CAD build for the part. Positions are in the model's coordinates, mm. Round coordinates to 2 decimals unless told otherwise and drop trailing zeros. Order: outer loops, then holes, each group sorted by start corner. A loop starts at its lowest first (then second) coordinate and runs counter-clockwise, first axis right, second up. Notation, with made-up numbers: (43, 42.25) - (52, 42.25) arc R24 ccw to (52, 64.25) - close; hole circle Ø10 at (31, -13.5). An arc over 180 degrees is marked (long way). Write item = value, one per line.
from build123d import *

# Parameters (mm, degrees)
SWEEP1_PROFILE_R    = 12.7
SKETCH2_R           = 25.4
BOSS_EXTRUDE1_DEPTH = 127
FILLET1_R           = 16.51


with BuildPart() as part:
    # Sweep1: sweep along a path in Sketch1
    with BuildLine(Plane.XY) as sweep1_path:
        Line((-127, 0), (-25.4, 0))
        ThreePointArc((-25.4, 0), (-7.439487758, 7.439487758), (0, 25.4))
        Line((0, 25.4), (0, 88.9))
    # Sweep1 profile (on start of the path) → Sweep1 (sweep)
    with BuildSketch(Plane.YZ.offset(-127)):
        Circle(SWEEP1_PROFILE_R)
    sweep(path=sweep1_path.line)

    # Sketch2 → Boss-Extrude1 (add)
    with BuildSketch(Plane(origin=(0, 88.9, 0), x_dir=(1, 0, 0), z_dir=(0, 1, 0))):
        with Locations(Location((0, 0, 0), (0, 0, 270))):
            Circle(SKETCH2_R)
    extrude(amount=BOSS_EXTRUDE1_DEPTH)

    # Fillet1
    # the kernel refuses this fillet: 16.51 mm, written as the material it takes off along each edge
    with BuildSketch(Plane(origin=(0, 88.9, 0), x_dir=(0, 0, 1), z_dir=(-1, 0, 0))) as fillet1_piece_1:
        with BuildLine():
            CenterArc((8.89, 16.064370514), FILLET1_R, 283.342363797, 76.657636203)
            Line((12.7, 0), (12.7762, -0.32128741))
            ThreePointArc((12.7762, -0.32128741), (19.05, -0.3302), (25.4, -0.3302))
            Line((25.4, -0.3302), (25.7302, 0))
            Line((25.7302, 0), (25.7302, 16.064370514))
            Line((25.7302, 16.064370514), (25.4, 16.064370514))
        make_face()
    revolve(axis=Axis((0, 88.9, 0), (0, 1, 0)), mode=Mode.SUBTRACT)


solid = part.part
(1) Probe line 1 along X through (y, z) = (140, -1); line 2 along Y through (x, z) = (-68.5, -1); line 3 along Y through (x, z) = (-69.5, 4). List the from-to ranges inside material, lowest first.
Solved:
line_1 = -25.38 to 25.38
line_2 = -12.66 to 12.66
line_3 = -12.05 to 12.05
(2) Drop flat-ended pins along their axis: pin 1 (5 mm diameter, centred on x = -63, z = 7, fed in from +Y); pin 2 (1.5 mm diameter, centred on x = -7.5, y = 160.5, fed in from +Z); pin 3 (2 mm diameter, centred on x = -45.5, z = 4, fed in from -Y). Give the stop position or say it passes through.
Solved:
pin_1 = 11.88
pin_2 = 24.49
pin_3 = -12.34
(3) Band-saw the part on B-B on x = -113. List the corners of the cut face in (y, z), plus the area to 3 significant figures.
Solved:
outline = circle Ø25.4 at (0, 0)
area = 507 mm²
(4) Band-saw the part on A-A on y = 112. List the corners of the cut face in (x, z).
Solved:
outline = circle Ø50.8 at (0, 0)
(5) Pull direction Y, two halves, no side cores. Call faces 1 (the cylindrical face through (-75.49, -2.75, -12.4)), 2 (the cylindrical face through (2.75, 57.59, -12.4)), 3 (the cylindrical face through (-15.456, 159.656, -20.157)): released by +Y, released by -Y, zero draft, split by the parting line, or undercut.
Solved:
face_1 = split by the parting line
face_2 = undercut
face_3 = zero draft
